Can you work these out from the model? Positions are in its coordinate system, mm. A direction names the side the tool comes from. Round coordinates to 2 decimals unless told otherwise and drop trailing zeros. Loops run counter-clockwise (first coordinate to the right, second up) from the corner with the lowest first, then second, coordinate; pieces in that order, holes last. Notation, with made-up numbers: M 13,-32 L 19,-32 A21 ccw 19,-12 Z; hole C 16.25,-12 d5. An arc over 180 degrees is marked long. Answer as CSV lines item,"result".
from build123d import *

# Parameters (mm, degrees)
F1_DEPTH = 76.2
F3_D     = 19.05
F5_D     = 19.05


with BuildPart() as f1:
    # F0 (on Front) → F1 (new body)
    with BuildSketch(Plane.XZ):
        Polygon((-31.7896687029, 19.3352506772), (-31.7896687029, -31.4647493228), (95.2103312971, -31.4647493228), (95.2103312971, -6.0647493228), (44.4103313356, -6.062771827), (44.0933883163, 19.3352506772), align=None)
    extrude(amount=F1_DEPTH)

    # F3 (through all)
    with Locations(Plane(origin=(44.3277707348, 0, 0.5531681646), x_dir=(0, 1, 0), z_dir=(0.9999221458, 0, 0.0124780716))):
        with Locations((-38.1, 6.0835448898)):
            Hole(F3_D / 2)

    # F5 (through all)
    with Locations(Plane.XY.offset(19.3352506772)):
        with Locations((6.1518598067, -38.1)):
            Hole(F5_D / 2)


solid = f1.part
Item 1: We'd pull the mould along Y, two halves only. Please class faces 1 (the face through (31, -38, -31.465)), 2 (the face through (-2.933, -35.239, -17.096)), 3 (the face through (17, 0, -11)), 4 (the face through (1.76, -46.55, 15.58)): released by +Y, released by -Y, zero draft, split by the parting line, or undercut.
Output:
face 1,"zero draft"
face 2,"undercut"
face 3,"released by +Y"
face 4,"undercut"
Item 2: On a 3-axis mill with a long thin cutter (end or side, diameter ignored), from which of +Z, -Z, +X, -X, +Y, -Y can I reach the whole of each face in a straight line? I mean faces 5 (the face through (-17.394, -28.584, 6.286)), 6 (the face through (17, -76.2, -11)). Say none if no direction works.
Output:
face 5,"none"
face 6,"+Z, -Z, +X, -X, -Y"
Item 3: If we section it at A-A on y = -38.1: Write out the boundary of the cut face in (x, z).
Output:
outline,"M -31.79,-31.46 L -3.37,-31.46 L -3.37,-3.48 L -31.79,-3.84 Z; M -31.79,15.21 L -3.37,15.57 L -3.37,19.34 L -31.79,19.34 Z; M 15.68,-31.46 L 95.21,-31.46 L 95.21,-6.06 L 44.41,-6.06 L 44.37,-2.89 L 15.68,-3.25 Z; M 15.68,15.81 L 44.13,16.16 L 44.09,19.34 L 15.68,19.34 Z"
Item 4: Will this pin go through, and if not, where does the flat tip stop? pin 1 (11.5 mm diameter, centred on x = 6.15, y = -38.1, fed in from -Z).
Output:
pin 1,"passes through"
Item 5: If we section it at C-C on y = -20.5: Write out the boundary of the cut face in (x, z), then the cut area to 3 significant figures.
Output:
outline,"M -31.79,-31.46 L 95.21,-31.46 L 95.21,-6.06 L 44.41,-6.06 L 44.09,19.34 L -31.79,19.34 Z"
area,"5,160 mm2"
Item 6: If we section it at B-B on z = -28: Write out the boundary of the cut face in (x, y) (3 decimals).
Output:
outline,"M -31.79,-76.2 L 95.21,-76.2 L 95.21,0 L -31.79,0 Z; hole C 6.152,-38.1 d19.05"
Item 7: If I drill on line 1 along X through (y, z) = (-39.5, -18.5); line 2 along X through (y, z) = (-38.1, -13); line 3 along Z through (x, y) = (87.5, -13), over which ranges is the centre line in solid material (lowest first)? Write a range as from..to.
Output:
line 1,"x = -31.79..-3.27, 15.57..95.21"
line 2,"x = -31.79..-3.37, 15.68..95.21"
line 3,"z = -31.46..-6.06"
